Part model, mm, in its own coordinate system. A direction names the side the tool comes from. Give positions to 0.01 mm unless a question says otherwise; leave off trailing zeros. Order: outer loops, then holes, each group sorted by start corner. A loop starts at its lowest first (then second) coordinate and runs counter-clockwise, first axis right, second up.
1. Slice it at B-B on y = 1.4. List the corners of the cut face in (x, z).
2. Slice it at A-A on x = 17.5. List the corners of the cut face in (y, z), and give its area (3 significant figures).
3. Drop flat-ended pins along their axis: pin 1 Ø6 at (x, z) = (27.5, 7.5) entering from -Y; pin 2 Ø3 at (x, y) = (26.5, -1) entering from -Z; pin 3 Ø6 at (x, z) = (10.5, 2) entering from +Y; pin 4 Ø2 at (x, z) = (24, -9) entering from +Y. Give the stop position or say it passes through.
4. Probe line 1 (Z direction, x = 59, y = 0.1); line 2 (Z direction, x = 3.5, y = 1.35); line 3 (Y direction, x = 34.5, z = -4.75). List the from-to ranges inside material, lowest first.
5. Which spindle directions (+Z, -Z, +X, -X, +Y, -Y) get a long thin tool onto all of the face, cutting with end or side? Do faces 1 (the flat face through (70, 0, -5)), 2 (the cylindrical face through (42.012, -0.751, 7.385)). Say none if no direction does.
from build123d import *

# Parameters (mm, degrees)
SKETCH_3_R = 2.5


with BuildPart() as part:
    # 扫描2: sweep along a path in 草图1
    with BuildLine(Plane(origin=(0, 0, 0), x_dir=(1, 0, 0), z_dir=(0, 1, 0))) as sweep_2_path:
        Line((70, 5), (13.228756555, 5))
        ThreePointArc((13.228756555, 5), (9.693222649, 5.645856533), (6.614378278, 7.5))
        ThreePointArc((6.614378278, 7.5), (-10, 0), (6.614378278, -7.5))
        ThreePointArc((6.614378278, -7.5), (9.693222649, -5.645856533), (13.228756555, -5))
        Line((13.228756555, -5), (70, -5))
    # 草图3 → 扫描2 (sweep)
    with BuildSketch(Plane(origin=(70, 0, 0), x_dir=(0, 0, -1), z_dir=(1, 0, 0))):
        with Locations((5, 0)):
            Circle(SKETCH_3_R)
    sweep(path=sweep_2_path.line)


solid = part.part
Data:
1. outline: (5.24, -5.95) arc R7.93 cw (long way) to (5.24, 5.95) arc R12.07 ccw to (13.23, 2.93) - (70, 2.93) - (70, 7.07) - (13.23, 7.07) arc R7.93 cw to (7.98, 9.05) arc R12.07 ccw (long way) to (7.98, -9.05) arc R7.93 cw to (13.23, -7.07) - (70, -7.07) - (70, -2.93) - (13.23, -2.93) arc R12.07 ccw to start
2. outline: circle Ø5 at (0, -5); circle Ø5 at (0, 5)
2. area: 39.3 mm2
3. pin 1: stops at y = -2.5
3. pin 2: stops at z = -7.5
3. pin 3: stops at y = 2.48
3. pin 4: passes through
4. line 1: z = -7.5 to -2.5, 2.5 to 7.5
4. line 2: z = -11.59 to -7.08, 7.08 to 11.59
4. line 3: y = -2.49 to 2.49
5. face 1: +Z, -Z, +X, +Y, -Y
5. face 2: +X
